Geometry: final body of the model. Coordinates: model frame, mm. Face numbers are marked on the shaded views. A direction names the side the tool comes from. Coordinates: 2 decimals unless noted, no trailing zeros. Write each loop counter-clockwise with the first axis right and the second up, starting at its lowest first coordinate (ties: lowest second). Pieces come first, ordered by that corner, then holes. Notation, with made-up numbers: (-14.75, 23.5) - (10.25, 23.5) arc R17 ccw to (10.25, 48.5) - close; hole circle Ø8 at (35.25, -7). An arc over 180 degrees is marked (long way). Put each result on its own line as item: value.
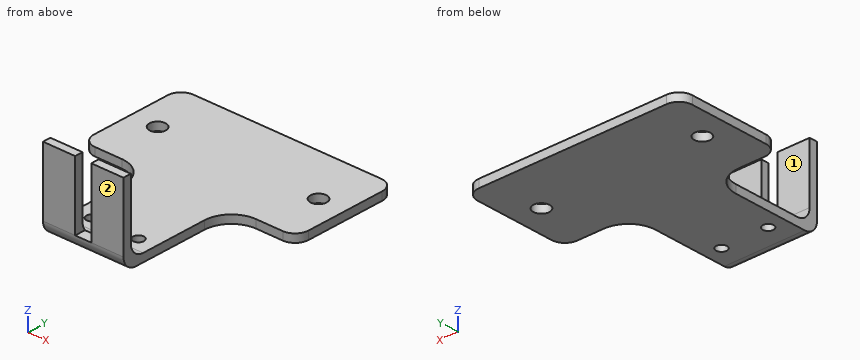
```python
from build123d import *

# Parameters (mm, degrees)
F1_DEPTH     = 3
F2_D         = 4
F3_D         = 6
F5_W         = 30
F5_H         = 3
F6_DEPTH     = 3
F7_T4_DEPTH  = 30
F7_T10_DEPTH = 30
F7_T16_DEPTH = 30
F7_T23_DEPTH = 30
F7_T29_DEPTH = 30
F7_T32_DEPTH = 55


# Not quite as in the source:
# - a fillet or chamfer that OpenCascade refuses, or shapes differently, is made with other operations: its cross-section is extruded or revolved along the edge and cut away or added


with BuildPart() as f1:
    # F0 (on Top) → F1 (new body)
    with BuildSketch(Plane.XY):
        with BuildLine():
            Line((40.0588317961, -2.3308048306), (-29.9411682039, -2.3308048306))
            ThreePointArc((-29.9411682039, -2.3308048306), (-33.4767021099, -3.7952709247), (-34.9411682039, -7.3308048306))
            Line((-34.9411682039, -7.3308048306), (-34.9411682039, -37.3308048306))
            ThreePointArc((-34.9411682039, -37.3308048306), (-33.4767021099, -40.8663387365), (-29.9411682039, -42.3308048306))
            Line((-29.9411682039, -42.3308048306), (-19.9411682039, -42.3308048306))
            ThreePointArc((-19.9411682039, -42.3308048306), (-12.8701003921, -45.2597370187), (-9.9411682039, -52.3308048306))
            Line((-9.9411682039, -52.3308048306), (-9.9411682039, -82.3308048306))
            Line((-9.9411682039, -82.3308048306), (5.0588317961, -82.3308048306))
            Line((5.0588317961, -82.3308048306), (20.0588317961, -82.3308048306))
            Line((20.0588317961, -82.3308048306), (20.0588317961, -52.3308048306))
            ThreePointArc((20.0588317961, -52.3308048306), (22.9877639842, -45.2597370187), (30.0588317961, -42.3308048306))
            Line((30.0588317961, -42.3308048306), (40.0588317961, -42.3308048306))
            ThreePointArc((40.0588317961, -42.3308048306), (43.594365702, -40.8663387365), (45.0588317961, -37.3308048306))
            Line((45.0588317961, -37.3308048306), (45.0588317961, -7.3308048306))
            ThreePointArc((45.0588317961, -7.3308048306), (43.594365702, -3.7952709247), (40.0588317961, -2.3308048306))
        make_face()
    extrude(amount=F1_DEPTH)

    # F2 (through all)
    with Locations(Plane(origin=(0, 0, 0), x_dir=(1, 0, 0), z_dir=(0, 0, -1))):
        with Locations((-3.6411682039, 72.3308048306), (13.7588317961, 72.3308048306)):
            Hole(F2_D / 2)

    # F3 (through all)
    with Locations(Plane(origin=(0, 0, 0), x_dir=(1, 0, 0), z_dir=(0, 0, -1))):
        with Locations((-24.9411682039, 22.3308048306), (35.0588317961, 22.3308048306)):
            Hole(F3_D / 2)

    # F5 (on face) → F6 (join)
    with BuildSketch(Plane.XZ.offset(82.3308048306)):
        Polygon((-9.9411682039, 30), (-9.9411682039, 3), (20.0588317961, 3), (20.0588317961, 30), (8.0588317961, 30), (8.0588317961, 5), (2.0588317961, 5), (2.0588317961, 30), align=None)
        with Locations((5.0588317961, 1.5)):
            Rectangle(F5_W, F5_H)
    extrude(amount=F6_DEPTH)

    # F7: fillet of radius 5 on 2 edges, made by hand


with BuildPart() as f7_tool2:
    # F7_s3 → F7_t4 (new body)
    with BuildSketch(Plane.YZ.offset(20.0588317961)):
        with BuildLine():
            ThreePointArc((-77.3308048306, 3), (-80.8663387365, 4.4644660941), (-82.3308048306, 8))
            Line((-82.3308048306, 8), (-82.3308048306, 3))
            Line((-82.3308048306, 3), (-77.3308048306, 3))
        make_face()
    extrude(amount=-F7_T4_DEPTH)

    split(bisect_by=Plane.XY.offset(5), keep=Keep.BOTTOM)

    split(bisect_by=Plane.YZ.offset(8.0588317961), keep=Keep.TOP)


with BuildPart() as f1_1:
    add(f1.part)

    # F7_t1: union F7_tool2
    add(f7_tool2.part)


with BuildPart() as f7_tool8:
    # F7_s9 → F7_t10 (new body)
    with BuildSketch(Plane.YZ.offset(20.0588317961)):
        with BuildLine():
            ThreePointArc((-77.3308048306, 3), (-80.8663387365, 4.4644660941), (-82.3308048306, 8))
            Line((-82.3308048306, 8), (-82.3308048306, 3))
            Line((-82.3308048306, 3), (-77.3308048306, 3))
        make_face()
    extrude(amount=-F7_T10_DEPTH)

    split(bisect_by=Plane.XY.offset(5), keep=Keep.TOP)

    split(bisect_by=Plane.YZ.offset(8.0588317961), keep=Keep.TOP)


with BuildPart() as f1_2:
    add(f1_1.part)

    # F7_t7: union F7_tool8
    add(f7_tool8.part)


with BuildPart() as f7_tool14:
    # F7_s15 → F7_t16 (new body)
    with BuildSketch(Plane.YZ.offset(20.0588317961)):
        with BuildLine():
            ThreePointArc((-77.3308048306, 3), (-80.8663387365, 4.4644660941), (-82.3308048306, 8))
            Line((-82.3308048306, 8), (-82.3308048306, 3))
            Line((-82.3308048306, 3), (-77.3308048306, 3))
        make_face()
    extrude(amount=-F7_T16_DEPTH)

    split(bisect_by=Plane.YZ.offset(2.0588317961), keep=Keep.TOP)

    split(bisect_by=Plane.XY.offset(5), keep=Keep.BOTTOM)

    split(bisect_by=Plane.YZ.offset(8.0588317961), keep=Keep.BOTTOM)


with BuildPart() as f1_3:
    add(f1_2.part)

    # F7_t13: union F7_tool14
    add(f7_tool14.part)


with BuildPart() as f7_tool21:
    # F7_s22 → F7_t23 (new body)
    with BuildSketch(Plane.YZ.offset(20.0588317961)):
        with BuildLine():
            ThreePointArc((-77.3308048306, 3), (-80.8663387365, 4.4644660941), (-82.3308048306, 8))
            Line((-82.3308048306, 8), (-82.3308048306, 3))
            Line((-82.3308048306, 3), (-77.3308048306, 3))
        make_face()
    extrude(amount=-F7_T23_DEPTH)

    split(bisect_by=Plane.YZ.offset(2.0588317961), keep=Keep.BOTTOM)

    split(bisect_by=Plane.XY.offset(5), keep=Keep.BOTTOM)


with BuildPart() as f1_4:
    add(f1_3.part)

    # F7_t20: union F7_tool21
    add(f7_tool21.part)


with BuildPart() as f7_tool27:
    # F7_s28 → F7_t29 (new body)
    with BuildSketch(Plane.YZ.offset(20.0588317961)):
        with BuildLine():
            ThreePointArc((-77.3308048306, 3), (-80.8663387365, 4.4644660941), (-82.3308048306, 8))
            Line((-82.3308048306, 8), (-82.3308048306, 3))
            Line((-82.3308048306, 3), (-77.3308048306, 3))
        make_face()
    extrude(amount=-F7_T29_DEPTH)

    split(bisect_by=Plane.YZ.offset(2.0588317961), keep=Keep.BOTTOM)

    split(bisect_by=Plane.XY.offset(5), keep=Keep.TOP)


with BuildPart() as f1_5:
    add(f1_4.part)

    # F7_t26: union F7_tool27
    add(f7_tool27.part)

    # F7_s33 → F7_t32 (cut)
    with BuildSketch(Plane.YZ.offset(-22.4411682039)):
        with BuildLine():
            ThreePointArc((-85.3308048306, 5), (-83.8663387365, 1.4644660941), (-80.3308048306, 0))
            Line((-80.3308048306, 0), (-85.3308048306, 0))
            Line((-85.3308048306, 0), (-85.3308048306, 5))
        make_face()
    extrude(amount=F7_T32_DEPTH, mode=Mode.SUBTRACT)


solid = f1_5.part
```
1. Section query B-B (x = 18.5). Return loops of the section in (y, z), then the cut area to 3 significant figures.
Answer below:
outline: (-85.33, 5) arc R5 ccw to (-80.33, 0) - (-2.33, 0) - (-2.33, 3) - (-77.33, 3) arc R5 cw to (-82.33, 8) - (-82.33, 30) - (-85.33, 30) - close
area: 330 mm²
2. Set-up query: the marked faces 1 and 2. Return all of +Z, -Z, +X, -X, +Y, -Y with unobstructed straight access to the full face (end or side cutting, diameter ignored); none if empty.
Answer below:
face 1: +Z, +X, -X, +Y
face 2: +Z, -Z, +X, -X, -Y
3. Section query D-D (y = -32.5). Return loops of the section in (x, z), then the cut area to 3 significant figures.
Answer below:
outline: (-34.94, 0) - (45.06, 0) - (45.06, 3) - (-34.94, 3) - close
area: 240 mm²
4. Section query A-A (z = 21.5). Return loops of the section in (x, y), then the cut area to 3 significant figures.
Answer below:
outline: (-9.94, -85.33) - (2.06, -85.33) - (2.06, -82.33) - (-9.94, -82.33) - close; (8.06, -85.33) - (20.06, -85.33) - (20.06, -82.33) - (8.06, -82.33) - close
area: 72.0 mm²
5. Ray query, probe 1 along Z at (x, y) = (-4.5, -14.5); probe 2 along Y at (x, z) = (18, 28); probe 3 along Y at (x, z) = (36.5, 2.5). Return the intervals inside material, ascending. Write a range as from..to.
Answer below:
probe 1: z = 0..3
probe 2: y = -85.33..-82.33
probe 3: y = -42.33..-24.96, -19.7..-2.33
6. Section query C-C (y = -56). Return loops of the section in (x, z).
Answer below:
outline: (-9.94, 0) - (20.06, 0) - (20.06, 3) - (-9.94, 3) - close
7. Pin query (flat end, axial travel): pin 1 Ø15 at (y, z) = (-66.5, 11) entering from +X; pin 2 Ø1.5 at (x, y) = (13, -13) entering from +Z; pin 3 Ø9.5 at (x, z) = (-5.5, 19) entering from +Y; pin 4 Ø4.5 at (x, y) = (5, -83.5) entering from +Z. Return the tip coordinate at first contact, or that it passes through.
Answer below:
pin 1: passes through
pin 2: stops at z = 3
pin 3: stops at y = -82.33
pin 4: stops at z = 5
